```python
from build123d import *

# Parameters (mm, degrees)
AUFSATZ_LINEAR_START            = 3
SKIZZE4_W                       = 100
SKIZZE4_H                       = 100
AUFSATZ_LINEAR_AUSTRAGEN1_DEPTH = 15


with BuildPart() as part:
    # Skizze4 → Aufsatz-Linear austragen1 (new body)
    with BuildSketch(Plane(origin=(0, 0, 0), x_dir=(1, 0, 0), z_dir=(0, 1, 0)).offset(AUFSATZ_LINEAR_START)):
        Rectangle(SKIZZE4_W, SKIZZE4_H)
    extrude(amount=-AUFSATZ_LINEAR_AUSTRAGEN1_DEPTH)

    # Schnitt-Austragung1: sweep along a path in Skizze1_2
    with BuildLine(Plane(origin=(0, 0, 0), x_dir=(1, 0, 0), z_dir=(0, 1, 0))) as schnitt_austragung1_path:
        Line((5, 0), (20, 0))
        ThreePointArc((20, 0), (35, -15), (20, -30))
        Line((20, -30), (-10, -30))
        ThreePointArc((-10, -30), (-17.071067812, -27.071067812), (-20, -20))
        Line((-20, -20), (-20, 0))
        ThreePointArc((-20, 0), (-15.867066806, 12.17522858), (-5.176380902, 19.318516526))
    # Skizze5 → Schnitt-Austragung1 (sweep, cut)
    with BuildSketch(Plane(origin=(0, 0, 0), x_dir=(-0.258819045, 0, -0.965925826), z_dir=(0.965925826, 0, -0.258819045))):
        with BuildLine():
            Line((21.1, 0), (21.1, 3))
            Line((21.1, 3), (18.9, 3))
            Line((18.9, 3), (18.9, 0))
            ThreePointArc((18.9, 0), (20, -1.1), (21.1, 0))
        make_face()
    sweep(path=schnitt_austragung1_path.line, mode=Mode.SUBTRACT)


solid = part.part
```
CAD build for the part. Positions are in the model's coordinates, mm. A direction names the side the tool comes from. Round coordinates to 2 decimals unless told otherwise and drop trailing zeros.
Item 1: Probe line 1 along Z through (x, y) = (-6, 0.75); line 2 along X through (y, z) = (1.25, -4.5); line 3 along Z through (x, y) = (-2, 2.25). List the from-to ranges inside material, lowest first.
Item 2: Tool access for faces 1 (the face through (-1, -4, 50)), 2 (the face through (-15.099, 1.479, -11.368)): list every direction of +Z, -Z, +X, -X, +Y, -Y with a clear straight run to the whole face (end or side of a thin tool).
Item 3: Mould opens along X. For faces 3 (the face through (50, -4, 1)), 4 (the face through (-20, -1.1, 9.9)), 5 (the face through (-1, -4, -50)) say: pulls with the +X half, pulls with the -X half, needs draft (parallel to the pull), parting line crosses it, or undercut.
Reported:
1. line 1: z = -50 to -20.23, -17.92 to 28.9, 31.1 to 50
1. line 2: x = -50 to -20.61, -18.36 to 50
1. line 3: z = -50 to 28.9, 31.1 to 50
2. face 1: +Z, +X, -X, +Y, -Y
2. face 2: +Y
3. face 3: pulls with the +X half
3. face 4: undercut
3. face 5: needs draft
